```python
from build123d import *

# Parameters (mm, degrees)
F0_R     = 6.5405
F0_R_2   = 3.048
F1_DEPTH = 25.4
F3_START = 25.4
F2_R     = 7.9375
F2_R_2   = 3.048
F3_DEPTH = 31.75
F4_SIZE  = 1.27


with BuildPart() as f1:
    # F0 (on Top) → F1 (new body)
    with BuildSketch(Plane.XY):
        Circle(F0_R)
        Circle(F0_R_2, mode=Mode.SUBTRACT)
    extrude(amount=F1_DEPTH)

    # F2 (on Top) → F3 (join)
    with BuildSketch(Plane.XY.offset(F3_START)):
        Circle(F2_R)
        Circle(F2_R_2, mode=Mode.SUBTRACT)
    extrude(amount=F3_DEPTH)

    # F4
    f4_edges = [f1.edges().sort_by_distance(p)[0] for p in [
        (-7.9375, 0, 57.15),
    ]]
    chamfer(f4_edges, length=F4_SIZE)


solid = f1.part
```
Input: part model. Units: mm. Frame: model coordinates. A direction names the side the tool comes from. Give positions to 0.01 mm unless a question says otherwise; leave off trailing zeros. Order: outer loops, then holes, each group sorted by start corner. A loop starts at its lowest first (then second) coordinate and runs counter-clockwise, first axis right, second up. Notation, with made-up numbers: M 2.25,57.25 L 32.25,57.25 A12 cw 32.25,79.25 Z; hole C 8,-18.75 d11. An arc over 180 degrees is marked long. Return JSON: item names as keys, results as strings.
1) Section query A-A on y = 0. Output: boundary loops of the cut face in (x, z), and give its area (3 significant figures).
Taken from the geometry:
{"outline": "M -7.94,25.4 L -6.54,25.4 L -6.54,0 L -3.05,0 L -3.05,57.15 L -6.67,57.15 L -7.94,55.88 Z; M 3.05,0 L 6.54,0 L 6.54,25.4 L 7.94,25.4 L 7.94,55.88 L 6.67,57.15 L 3.05,57.15 Z", "area": "486 mm2"}
2) Section query D-D on z = 19.5. Output: boundary loops of the cut face in (x, y), and give its area (3 significant figures).
Taken from the geometry:
{"outline": "C 0,0 d13.08; hole C 0,0 d6.1", "area": "105 mm2"}
3) Access query for faces 1 (the face through (3, 2, 0)), 2 (the face through (1, 7, 25.4)). Directions: +Z, -Z, +X, -X, +Y, -Y. A direction counts if a zero-diameter tool reaches every point of the face in a straight line with its end or side. Return the directions, or none.
Taken from the geometry:
{"face 1": "-Z, +X, -X, +Y, -Y", "face 2": "-Z"}
4) Contact query for flat-ended pins moving along their axis: pin 1 (3 mm diameter, centred on y = 6, z = 30, fed in from +X); pin 2 (5 mm diameter, centred on x = 2, z = 16.5, fed in from +Y); pin 3 (4 mm diameter, centred on x = 4.5, z = 49.5, fed in from -Y). Output: stop coordinate, or through.
Taken from the geometry:
{"pin 1": "stops at x = 6.54", "pin 2": "stops at y = 6.54", "pin 3": "stops at y = -7.53"}
5) Section query C-C on z = 47. Output: boundary loops of the cut face in (x, y) (1 decimal), and give its area (3 significant figures).
Taken from the geometry:
{"outline": "C 0,0 d15.9; hole C 0,0 d6.1", "area": "169 mm2"}
6) Line query: L1, parallel to Y at x = 0, z = 35; L2, parallel to Y at x = 0, z = 18.5; L3, parallel to X at y = 2, z = 26. Output: solid intervals per line, ascending. Write a range as [from, to].
Taken from the geometry:
{"L1": "y = [-7.94, -3.05], [3.05, 7.94]", "L2": "y = [-6.54, -3.05], [3.05, 6.54]", "L3": "x = [-7.68, -2.3], [2.3, 7.68]"}
7) Mould query, pull axis X, two halves, no side actions, for faces 3 (the face through (-0.4, 3.02, 28.17)), 4 (the face through (-0.851, 6.485, 12.522)), 5 (the face through (2.9, -1.4, 57.15)). Classes: released by +X, released by -X, zero draft, split by the parting line, or undercut.
Taken from the geometry:
{"face 3": "undercut", "face 4": "split by the parting line", "face 5": "zero draft"}
